from build123d import *

# Parameters (mm, degrees)
BOSS_EXTRUDE1_DEPTH = 34
SKETCH2_R           = 20
BOSS_EXTRUDE2_DEPTH = 2
SKETCH3_R           = 17.5
BOSS_EXTRUDE3_DEPTH = 5
SKETCH4_R           = 15
BOSS_EXTRUDE4_DEPTH = 5
SKETCH5_R           = 12
CUT_EXTRUDE1_DEPTH  = 5
CUT_EXTRUDE2_DEPTH  = 5
SKETCH10_W          = 3.955735376
SKETCH10_H          = 3.547567536
BOSS_EXTRUDE5_DEPTH = 5


with BuildPart() as part:
    # Sketch1 → Boss-Extrude1 (new body)
    with BuildSketch(Plane.XY):
        with BuildLine():
            Line((86, 5.125978653), (86, 34.874021347))
            ThreePointArc((86, 34.874021347), (84.803408431, 39.617437837), (81.5, 43.225667891))
            ThreePointArc((81.5, 43.225667891), (43, 54.764142081), (4.5, 43.225667891))
            ThreePointArc((4.5, 43.225667891), (1.196591569, 39.617437837), (0, 34.874021347))
            Line((0, 34.874021347), (0, 5.125978653))
            ThreePointArc((0, 5.125978653), (1.196591569, 0.382562163), (4.5, -3.225667891))
            ThreePointArc((4.5, -3.225667891), (43, -14.764142081), (81.5, -3.225667891))
            ThreePointArc((81.5, -3.225667891), (84.803408431, 0.382562163), (86, 5.125978653))
        make_face()
    extrude(amount=BOSS_EXTRUDE1_DEPTH)

    # Sketch2 → Boss-Extrude2 (add)
    with BuildSketch(Plane.XY.offset(34)):
        with Locations((43, 20)):
            Circle(SKETCH2_R)
    extrude(amount=BOSS_EXTRUDE2_DEPTH)

    # Sketch3 → Boss-Extrude3 (add)
    with BuildSketch(Plane.XY.offset(36)):
        with Locations((43, 20)):
            Circle(SKETCH3_R)
    extrude(amount=BOSS_EXTRUDE3_DEPTH)

    # Sketch4 → Boss-Extrude4 (add)
    with BuildSketch(Plane.XY.offset(41)):
        with Locations((43, 20)):
            Circle(SKETCH4_R)
    extrude(amount=BOSS_EXTRUDE4_DEPTH)

    # Sketch5 → Cut-Extrude1 (cut)
    with BuildSketch(Plane.XY.offset(46)):
        with Locations((43, 20)):
            Circle(SKETCH5_R)
    extrude(amount=-CUT_EXTRUDE1_DEPTH, mode=Mode.SUBTRACT)

    # Sketch9 → Cut-Extrude2 (cut)
    with BuildSketch(Plane(origin=(0, -14.764142081, 0), x_dir=(-1, 0, 0), z_dir=(0, -1, 0))):
        Polygon((-43, -13.35), (-47.25, -13.35), (-47.25, -19.65), (-46.25, -20.65), (-43, -20.65), (-39.75, -20.65), (-38.75, -19.65), (-38.75, -13.35), align=None)
    extrude(amount=-CUT_EXTRUDE2_DEPTH, mode=Mode.SUBTRACT)

    # Sketch10 → Boss-Extrude5 (add)
    with BuildSketch(Plane(origin=(0, -9.764142081, 0), x_dir=(-1, 0, 0), z_dir=(0, -1, 0))):
        with Locations((-43, -17)):
            Rectangle(SKETCH10_W, SKETCH10_H)
    extrude(amount=BOSS_EXTRUDE5_DEPTH)


solid = part.part
Model file for the job. Use its own axes, mm. A direction names the side the tool comes from. Round coordinates to 2 decimals unless told otherwise and drop trailing zeros. Loops run counter-clockwise (first coordinate to the right, second up) from the corner with the lowest first, then second, coordinate; pieces in that order, holes last. Notation, with made-up numbers: M 89,17 L 101,17 A18 ccw 101,42 Z; hole C -12,-28.75 d6. An arc over 180 degrees is marked long. One line per question, with ' | ' between items.
1) Band-saw the part on A-A (z = 12). Give the cut face in (x, y), then the cut area to 3 significant figures.
Solved:
outline: M 0,5.13 A10 ccw 4.5,-3.23 A70 ccw 81.5,-3.23 A10 ccw 86,5.13 L 86,34.87 A10 ccw 81.5,43.23 A70 ccw 4.5,43.23 A10 ccw 0,34.87 Z | area: 5,160 mm²
2) Drill centre lines: line 1 along Y through (x, z) = (43, 44.2); line 2 along Z through (x, y) = (51, 43); line 3 along Y through (x, z) = (44, 32). Where is each one in solid material? Low to high.
Solved:
line 1: y = 5 to 8, 32 to 35 | line 2: z = 0 to 34 | line 3: y = -14.76 to 54.76
3) Band-saw the part on B-B (x = 43). Give the cut face in (y, z).
Solved:
outline: M -14.76,0 L 54.76,0 L 54.76,34 L 40,34 L 40,36 L 37.5,36 L 37.5,41 L 35,41 L 35,46 L 32,46 L 32,41 L 8,41 L 8,46 L 5,46 L 5,41 L 2.5,41 L 2.5,36 L 0,36 L 0,34 L -14.76,34 L -14.76,20.65 L -9.76,20.65 L -9.76,18.77 L -14.76,18.77 L -14.76,15.23 L -9.76,15.23 L -9.76,13.35 L -14.76,13.35 Z
4) Flat gauge pins, fed straight in: pin 1 (1.5 mm diameter, centred on x = 52.5, z = 33.5, fed in from +Y); pin 2 (1.5 mm diameter, centred on x = 44, y = -13, fed in from +Z); pin 3 (5.5 mm diameter, centred on y = -12.5, z = 17.5, fed in from +X); pin 4 (4 mm diameter, centred on x = 75.5, y = 31.5, fed in from -Z). Where does each tip first touch, or does it go through?
Solved:
pin 1: stops at y = 54.22 | pin 2: stops at z = 34 | pin 3: stops at x = 69.02 | pin 4: stops at z = 0
5) Band-saw the part on C-C (y = 20). Give the cut face in (x, z), then the cut area to 3 significant figures.
Solved:
outline: M 0,0 L 86,0 L 86,34 L 63,34 L 63,36 L 60.5,36 L 60.5,41 L 58,41 L 58,46 L 55,46 L 55,41 L 31,41 L 31,46 L 28,46 L 28,41 L 25.5,41 L 25.5,36 L 23,36 L 23,34 L 0,34 Z | area: 3,210 mm²
6) 3-axis set-ups, long thin cutter, end or side, ignore diameter. For faces 1 (the flat face through (43, -12, 15.226)), 2 (the cylindrical face through (33.477, 12.698, 43.535)), 3 (the cylindrical face through (1.23, 39.68, 16.76)): which of +Z, -Z, +X, -X, +Y, -Y reach the whole face in a straight line?
Solved:
face 1: -Y | face 2: +Z | face 3: +Z, -Z, -X, +Y
7) Mould opens along Z. For faces 4 (the flat face through (44.978, -12, 17)), 5 (the flat face through (86, 20, 17)), 6 (the flat face through (42, 20, 0)) say: +Z half, -Z half, draft (parallel to the pull), parting line (faces both ways), or undercut.
Solved:
face 4: undercut | face 5: draft | face 6: -Z half
8) Band-saw the part on D-D (x = 32). Give the cut face in (y, z).
Solved:
outline: M -13.89,0 L 53.89,0 L 53.89,34 L 36.7,34 L 36.7,36 L 33.61,36 L 33.61,41 L 30.2,41 L 30.2,46 L 24.8,46 L 24.8,41 L 15.2,41 L 15.2,46 L 9.8,46 L 9.8,41 L 6.39,41 L 6.39,36 L 3.3,36 L 3.3,34 L -13.89,34 Z
